Work out the finished part from the listing and answer in its coordinate system (mm). A direction names the side the tool comes from. Round coordinates to 2 decimals unless told otherwise and drop trailing zeros. Answer as a JSON object with one key per item and string values. Group by question number.
Autodesk Inventor part; units mm, degrees
ref_plane "YZ Plane" through (0, 0, 0) normal (1, 0, 0) x (0, 1, 0)
ref_plane "XZ Plane" through (0, 0, 0) normal (0, 1, 0) x (-1, 0, 0)
ref_plane "XY Plane" through (0, 0, 0) normal (0, 0, 1) x (1, 0, 0)
sketch "Sketch1" plane through (0, 0, 0) normal (0, 1, 0) x (-1, 0, 0)
  circle A0 centre (0, 0) radius 28.575
  dimension "d0" = 57.15
extrude "Extrusion1" add sketch "Sketch1" along normal blind 0.7937
sketch "Sketch2" plane through (0, 0.7937, 0) normal (0, 1, 0) x (1, 0, 0)
  line L0 (0, 0) -> (-28.575, 0) construction
  circle A0 centre (0, 0) radius 28.575
  line L1 (-6.35, 0) -> (-3.175, 5.4993)
  line L2 (-3.175, 5.4993) -> (3.175, 5.4993)
  line L3 (3.175, 5.4993) -> (6.35, 0)
  line L4 (6.35, 0) -> (3.175, -5.4993)
  line L5 (3.175, -5.4993) -> (-3.175, -5.4993)
  line L6 (-3.175, -5.4993) -> (-6.35, 0)
  circle A1 centre (0, 0) radius 23.8125
  circle A2 centre (0, 0) radius 24.6063
  circle A3 centre (0, 0) radius 27.7812
  circle A4 centre (0, 0) radius 7.5565
  circle A5 centre (0, 0) radius 12.7 construction
  circle A6 centre (-12.7, 0) radius 1.7526
  circle A7 centre (-6.35, -10.9985) radius 1.7526
  circle A8 centre (6.35, -10.9985) radius 1.7526
  circle A9 centre (12.7, 0) radius 1.7526
  circle A10 centre (6.35, 10.9985) radius 1.7526
  circle A11 centre (-6.35, 10.9985) radius 1.7526
  dimension "d18" = 25.4
  dimension "d3" = 6.35
  dimension "d4" = 47.625
  dimension "d5" = 0.7937
  dimension "d6" = 0.7937
  dimension "d15" = 15.113
  dimension "d19" = 3.5052
  dimension "d22" = 360
extrude "Extrusion2" add sketch "Sketch2" along normal blind 8.89 contours L1 L2 L3 L4 L5 L6 | A2
fillet "Fillet1" radius 0.508 6 edges at (6.35, 5.2387, 0) (3.175, 5.2387, -5.4993) (-3.175, 5.2387, -5.4993) (-6.35, 5.2387, 0) (-3.175, 5.2387, 5.4993) (3.175, 5.2387, 5.4993)
extrude "Extrusion3" add sketch "Sketch2" along normal blind 12.7 contours A0
chamfer "Chamfer1" distance 0.7937 angle 45 1 edges at (-23.8125, 0.7937, 0)
extrude "Extrusion4" add sketch "Sketch2" along normal blind 1.27 contours L1 L2 L3 L4 L5 L6 | A4
extrude "Extrusion5" cut sketch "Sketch2" against normal through all contours A6 | A7 | A8 | A9 | A10 | A11
sketch "Sketch3" plane through (0, 9.6837, 0) normal (0, 1, 0) x (1, 0, 0)
  circle A0 centre (0, 0) radius 1.7526
  dimension "d26" = 3.5052
extrude "Extrusion6" cut sketch "Sketch3" against normal through all
properties part number "Wheel V2 Mold"
Item 1: The mould has two halves that part along Z. Classify faces 1 (the flat face through (-6, 0, 0)), 2 (the cylindrical face through (4.959, 0.402, 12.065)): +Z half, -Z half, draft (parallel to the pull), parting line (faces both ways), or undercut.
Item 2: Each of these flat-tipped pins is pushed along its axis until it touches: pin 1 (4 mm diameter, centred on x = -1.5, z = -13, fed in from +Y); pin 2 (3 mm diameter, centred on x = -1, y = 4, fed in from +Z) (3 decimals); pin 3 (8 mm diameter, centred on y = 3, z = -12, fed in from -X). Where does it stop, or does it pass through?
Item 3: Consider L1, parallel to X at y = 8, z = 0 (1 decimal); L2, parallel to X at y = 0.25, z = 0 (3 decimals); L3, parallel to Z at x = -6.35, y = 0.6. Determine where each line is inside the solid, lowest interval first.
Item 4: A tool of negligible diameter and unlimited length cuts with its end or side. For faces 3 (the cylindrical face through (-3.203, 5.176, 24.397)), 4 (the flat face through (-4, 13.494, -28)), from which of +Z, -Z, +X, -X, +Y, -Y can it reach the whole face along a straight path? Write none if from no direction.
Item 5: Find section A-A (y = 4). Give the number of separate pieces and of enclosed holes in the cut face, and give its area (3 significant figures).
Responses:
{
 "1": {"face 1": "draft", "face 2": "undercut"},
 "2": {"pin 1": "stops at y = 0.79", "pin 2": "stops at z = 28.575", "pin 3": "stops at x = -27.43"},
 "3": {"L1": "x = -28.6 to -27.8, -24.6 to -23.8, -6.3 to -1.8, 1.8 to 6.3, 23.8 to 24.6, 27.8 to 28.6", "L2": "x = -28.575 to -14.453, -10.947 to -1.753, 1.753 to 10.947, 14.453 to 28.575", "L3": "z = -27.86 to -12.75, -9.25 to 9.25, 12.75 to 27.86"},
 "4": {"face 3": "+Y", "face 4": "+Z, -Z, +X, -X, +Y"},
 "5": {"separate pieces": "3", "enclosed holes": "3", "area": "356 mm^2"}
}
